```python
from build123d import *

# Parameters (mm, degrees)
F0_W     = 63.5
F0_H     = 38.1
F1_DEPTH = 22.225
F2_R     = 3.96875
F3_DEPTH = 4.445
F4_R     = 2.38125
F5_DEPTH = 33.656


with BuildPart() as f1:
    # F0 (on Front) → F1 (new body, symmetric)
    with BuildSketch(Plane.XZ):
        Rectangle(F0_W, F0_H)
    extrude(amount=F1_DEPTH, both=True)

    # F2 (on face) → F3 (cut)
    with BuildSketch(Plane.XY.offset(19.05)):
        Circle(F2_R)
    extrude(amount=-F3_DEPTH, mode=Mode.SUBTRACT)

    # F4 (on face) → F5 (cut, through all)
    with BuildSketch(Plane.XY.offset(14.605)):
        Circle(F4_R)
    extrude(amount=-F5_DEPTH, mode=Mode.SUBTRACT)


solid = f1.part
```
Geometry check sheet. Reference: the model listing, model coordinates, mm. A direction names the side the tool comes from. Coordinates: 2 decimals unless noted, no trailing zeros. Order: outer loops, then holes, each group sorted by start corner. A loop starts at its lowest first (then second) coordinate and runs counter-clockwise, first axis right, second up. Notation, with made-up numbers: M -15.5,-5.75 L 21.5,-5.75 A11 ccw 21.5,6.25 Z; hole C 17,79.25 d4. An arc over 180 degrees is marked long. One line per question, with ' | ' between items. Start each with the question number.
Item 1: Cross-section at B-B on y = 0. Enter the section's corners in (x, z) (3 decimals).
Item 2: Material ranges on L1, parallel to Y at x = 0, z = -8 (3 decimals); L2, parallel to Y at x = 0, z = 17.8 (3 decimals), recorded low to high. Write a range as [from, to].
Item 3: Set-up check for faces 1 (the cylindrical face through (-1.89, -1.45, -1.99)), 2 (the cylindrical face through (-0.86, -3.874, 16.859)): record each of +Z, -Z, +X, -X, +Y, -Y from which the full face is reachable in a straight line by a thin tool's end or side.
Item 4: Cross-section at A-A on x = 0. Enter the section's corners in (y, z) (3 decimals), then the cut area to 3 significant figures.
Item 5: Gauge pin test, flat ends, axial feed: pin 1 (6.5 mm diameter, centred on x = 1.5, y = 2, fed in from +Z); pin 2 (5 mm diameter, centred on x = 0, y = 0, fed in from +Z) (3 decimals). Record the tip position at first contact, or that the pin passes through.
Item 6: Draft check along X on faces 3 (the flat face through (2, -2, 14.605)), 4 (the flat face through (-31.75, 0, 0)), 5 (the flat face through (0, -5, 19.05)). Enter one of: pulls with the +X half, pulls with the -X half, needs draft (parallel to the pull), parting line crosses it, or undercut.
Findings:
1) outline: M -31.75,-19.05 L -2.381,-19.05 L -2.381,14.605 L -3.969,14.605 L -3.969,19.05 L -31.75,19.05 Z; M 2.381,-19.05 L 31.75,-19.05 L 31.75,19.05 L 3.969,19.05 L 3.969,14.605 L 2.381,14.605 Z
2) L1: y = [-22.225, -2.381], [2.381, 22.225] | L2: y = [-22.225, -3.969], [3.969, 22.225]
3) face 1: +Z, -Z | face 2: +Z
4) outline: M -22.225,-19.05 L -2.381,-19.05 L -2.381,14.605 L -3.969,14.605 L -3.969,19.05 L -22.225,19.05 Z; M 2.381,-19.05 L 22.225,-19.05 L 22.225,19.05 L 3.969,19.05 L 3.969,14.605 L 2.381,14.605 Z | area: 1,500 mm²
5) pin 1: stops at z = 19.05 | pin 2: stops at z = 14.605
6) face 3: undercut | face 4: pulls with the -X half | face 5: needs draft
